Verification items for the finished model (mm, model axes). A direction names the side the tool comes from. Give positions to 0.01 mm unless a question says otherwise; leave off trailing zeros. Loops run counter-clockwise (first coordinate to the right, second up) from the corner with the lowest first, then second, coordinate; pieces in that order, holes last. Notation, with made-up numbers: M 53,23.25 L 103,23.25 A15 ccw 103,32.25 Z; hole C 15.5,32.5 d5. An arc over 180 degrees is marked long. Use a Markdown table: item, result.
Autodesk Inventor part; units mm, degrees
ref_plane "YZ Plane" through (0, 0, 0) normal (1, 0, 0) x (0, 1, 0)
ref_plane "XZ Plane" through (0, 0, 0) normal (0, 1, 0) x (-1, 0, 0)
ref_plane "XY Plane" through (0, 0, 0) normal (0, 0, 1) x (1, 0, 0)
sketch "Sketch1" plane through (0, 0, 0) normal (0, 0, 1) x (1, 0, 0)
  circle A0 centre (0, 0) radius 6.477
  dimension "d0" = 12.954
extrude "Extrusion1" add sketch "Sketch1" against normal blind 282.575
sketch "Sketch3" plane through (0, 0, 0) normal (0, 1, 0) x (-1, 0, 0)
  line L0 (-6.477, -282.575) -> (6.477, -282.575)
  line L1 (-6.477, 0) -> (6.477, 0)
  line L2 (6.477, 0) -> (6.477, -282.575)
  line L3 (-6.477, 0) -> (-6.477, -282.575)
  line L4 (0, 0) -> (0, 36.576)
  line L5 (5.1435, 36.576) -> (5.1435, 6.096)
  line L6 (0, 36.576) -> (5.1435, 36.576)
  line L7 (5.1435, 6.096) -> (6.477, 0)
  line L8 (6.477, 0) -> (0, 0)
  dimension "d3" = 36.576
  dimension "d4" = 5.1435
  dimension "d5" = 30.48
revolve "Revolution1" add sketch "Sketch3" angle 360 about axis through (0, 0, 0) along (0, 0, 1) contours L1 L4 L6 L5 L7
sketch "Sketch4" plane through (0, 0, 36.576) normal (0, 0, 1) x (1, 0, 0)
  circle A0 centre (0, 0) radius 5.1435
  circle A1 centre (0, 0) radius 3.6957
  dimension "d7" = 7.3914
extrude "Extrusion2" cut sketch "Sketch4" against normal blind 36.576 contours A1
sketch "Sketch5" plane through (0, 0, -282.575) normal (0, 0, -1) x (-1, 0, 0)
  circle A0 centre (0, 0) radius 6.477
  circle A1 centre (0, 0) radius 5.1562
  dimension "d10" = 10.3124
extrude "Extrusion3" cut sketch "Sketch5" against normal blind 282.702 contours A1
properties part number "Cane Segment"
(1) Material ranges on line 1 (Y direction, x = 0, z = 24); line 2 (Y direction, x = 0, z = -167.5); line 3 (Z direction, x = -3.5, y = -2.5), recorded low to high.
Results below:
| item | result |
|---|---|
| line 1 | -5.14 to -3.7, 3.7 to 5.14 |
| line 2 | -6.48 to -5.16, 5.16 to 6.48 |
| line 3 | 0.13 to 36.58 |
(2) Cross-section at D-D on z = 12.5. Record the cut outline in (x, y), then the cut area to 3 significant figures.
Results below:
| item | result |
|---|---|
| outline | C 0,0 d10.29; hole C 0,0 d7.39 |
| area | 40.2 mm^2 |
(3) Cross-section at A-A on y = 0. Record the cut outline in (x, z) (1 decimal), then the cut area to 3 significant figures.
Results below:
| item | result |
|---|---|
| outline | M -6.5,-282.6 L -5.2,-282.6 L -5.2,0.1 L -3.7,0.1 L -3.7,36.6 L -5.1,36.6 L -5.1,6.1 L -6.5,0 Z; M 3.7,0.1 L 5.2,0.1 L 5.2,-282.6 L 6.5,-282.6 L 6.5,0 L 5.1,6.1 L 5.1,36.6 L 3.7,36.6 Z |
| area | 860 mm^2 |
(4) Cross-section at C-C on z = -28. Record the cut outline in (x, y).
Results below:
| item | result |
|---|---|
| outline | C 0,0 d12.95; hole C 0,0 d10.31 |
(5) Draft check along X on faces 1 (the cylindrical face through (-1.404, -6.323, -139.309)), 2 (the flat face through (1, -4, 36.576)), 3 (the flat face through (1, 4, 0.127)). Enter one of: +X half, -X half, draft (parallel to the pull), parting line (faces both ways), or undercut.
Results below:
| item | result |
|---|---|
| face 1 | parting line |
| face 2 | draft |
| face 3 | undercut |
(6) Gauge pin test, flat ends, axial feed: P1, Ø6, axis at y = -1, z = -160, coming from the +X side; P2, Ø5, axis at x = -3.5, z = -52, coming from the -Y side; P3, Ø1.5, axis at y = -2.5, z = -67.5, coming from the -X side; P4, Ø5, axis at y = -4.5, z = -66.5, coming from the +X side. Record the tip position at first contact, or that the pin passes through.
Results below:
| item | result |
|---|---|
| P1 | x = 6.48 |
| P2 | y = -6.4 |
| P3 | x = -6.24 |
| P4 | x = 6.16 |
(7) Set-up check for faces 4 (the cylindrical face through (-0.8, -3.61, 18.61)), 5 (the cylindrical face through (0.67, 5.1, 21.12)), 6 (the cylindrical face through (-2.77, 4.35, -143.2)): record each of +Z, -Z, +X, -X, +Y, -Y from which the full face is reachable in a straight line by a thin tool's end or side.
Results below:
| item | result |
|---|---|
| face 4 | +Z, -Z |
| face 5 | +Z |
| face 6 | -Z |
